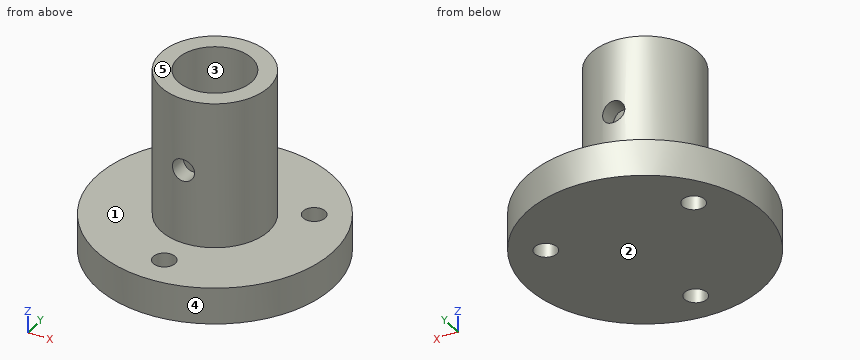
from build123d import *

# Parameters (mm, degrees)
SKETCH1_R               = 32
SKETCH1_R_2             = 3
BOSS_EXTRUDE1_DEPTH     = 9.9
SKETCH2_R               = 14.6
SKETCH2_R_2             = 10
BOSS_EXTRUDE2_DEPTH     = 39.8
SKETCH3_R               = 3
CUT_EXTRUDE1_DEPTH      = 33
CUT_EXTRUDE1_DEPTH_BACK = 33


with BuildPart() as part:
    # Sketch1 → Boss-Extrude1 (new body)
    with BuildSketch(Plane.XY):
        Circle(SKETCH1_R)
        with Locations((20, 11.547005384)):
            Circle(SKETCH1_R_2, mode=Mode.SUBTRACT)
        with Locations((0, -23.094010768)):
            Circle(SKETCH1_R_2, mode=Mode.SUBTRACT)
        with Locations((-20, 11.547005384)):
            Circle(SKETCH1_R_2, mode=Mode.SUBTRACT)
    extrude(amount=BOSS_EXTRUDE1_DEPTH)

    # Sketch2 → Boss-Extrude2 (add)
    with BuildSketch(Plane.XY.offset(9.9)):
        Circle(SKETCH2_R)
        Circle(SKETCH2_R_2, mode=Mode.SUBTRACT)
    extrude(amount=BOSS_EXTRUDE2_DEPTH)

    # Sketch3 → Cut-Extrude1 (cut, two sides)
    with BuildSketch(Plane(origin=(0, 0, 0), x_dir=(1, 0, 0), z_dir=(0, 1, 0))) as cut_extrude1_sk:
        with Locations((0, -30.05)):
            Circle(SKETCH3_R)
    extrude(amount=CUT_EXTRUDE1_DEPTH, mode=Mode.SUBTRACT)
    extrude(cut_extrude1_sk.sketch, amount=-CUT_EXTRUDE1_DEPTH_BACK, mode=Mode.SUBTRACT)


solid = part.part
Source: CAD feature listing. Evaluate the final solid. Frame: model axes, mm. Face numbers are marked on the shaded views. A direction names the side the tool comes from. Round coordinates to 2 decimals unless told otherwise and drop trailing zeros. Loops run counter-clockwise (first coordinate to the right, second up) from the corner with the lowest first, then second, coordinate; pieces in that order, holes last.
Q1. First-contact query: P1, Ø5, axis at y = -8.5, z = 33, coming from the +X side; P2, Ø8, axis at x = 20, y = 11.55, coming from the +Z side; P3, Ø1.5, axis at y = -0.5, z = 34.5, coming from the +X side. Flat tips, straight axial feed; report the tip coordinate or a pass-through.
Q2. Mould query, pull axis X, two halves, no side actions, for the marked faces 3, 4 and 5. Classes: pulls with the +X half, pulls with the -X half, needs draft (parallel to the pull), parting line crosses it, or undercut.
Q3. Access query for the marked faces 1 and 2. Directions: +Z, -Z, +X, -X, +Y, -Y. A direction counts if a zero-diameter tool reaches every point of the face in a straight line with its end or side. Return the directions, or none.
Q4. Section B-B, the plane x = 0. Return loops of the section in (y, z).
Q5. Section D-D, the plane z = 14. Return loops of the section in (x, y), plus the area to 3 significant figures.
Q6. Ray query, line 1 (Z direction, x = 0, y = 12); line 2 (Y direction, x = 0, z = 36); line 3 (Z direction, x = -12.5, y = 19.5). Return the intervals inside material, ascending.
Q7. Section A-A, the plane x = 20. Return loops of the section in (y, z).
Q8. Section C-C, the plane y = -11.5. Return loops of the section in (x, z) (3 decimals).
Solutions:
1. P1: stops at x = 13.31
1. P2: stops at z = 9.9
1. P3: stops at x = 14.6
2. face 3: undercut
2. face 4: parting line crosses it
2. face 5: needs draft
3. face 1: +Z
3. face 2: -Z, +X, -X, +Y, -Y
4. outline: (-32, 0) - (-26.09, 0) - (-26.09, 9.9) - (-32, 9.9) - close; (-20.09, 0) - (32, 0) - (32, 9.9) - (14.6, 9.9) - (14.6, 27.05) - (10, 27.05) - (10, 9.9) - (-10, 9.9) - (-10, 27.05) - (-14.6, 27.05) - (-14.6, 9.9) - (-20.09, 9.9) - close; (-14.6, 33.05) - (-10, 33.05) - (-10, 49.7) - (-14.6, 49.7) - close; (10, 33.05) - (14.6, 33.05) - (14.6, 49.7) - (10, 49.7) - close
5. outline: circle Ø29.2 at (0, 0); hole circle Ø20 at (0, 0)
5. area: 356 mm2
6. line 1: z = 0 to 27.05, 33.05 to 49.7
6. line 2: y = -14.6 to -10, 10 to 14.6
6. line 3: z = 0 to 9.9
7. outline: (-24.98, 0) - (8.55, 0) - (8.55, 9.9) - (-24.98, 9.9) - close; (14.55, 0) - (24.98, 0) - (24.98, 9.9) - (14.55, 9.9) - close
8. outline: (-29.862, 0) - (29.862, 0) - (29.862, 9.9) - (8.995, 9.9) - (8.995, 49.7) - (-8.995, 49.7) - (-8.995, 9.9) - (-29.862, 9.9) - close; hole circle Ø6 at (0, 30.05)
